Autodesk Inventor part; units mm, degrees
ref_plane "Startebene" through (0, 0, 0) normal (0, 0, 1) x (1, 0, 0)
ref_plane "Endebene" through (0, 0, 50) normal (0, 0, 1) x (1, 0, 0)
ref_plane "YZ Plane" through (0, 0, 0) normal (1, 0, 0) x (0, 1, 0)
ref_plane "Startebene" through (0, 0, 0) normal (0, 0, 1) x (1, 0, 0)
ref_plane "Endebene" through (0, 0, 50) normal (0, 0, 1) x (1, 0, 0)
sketch "Skizze2" plane through (0, 0, 0) normal (0, 0, 1) x (1, 0, 0)
  line L0 (-13.1, -4.1) -> (-13.1, 45.9)
  line L1 (-19.1, 50.9) -> (-18.1, 50.9)
  line L2 (-19.1, -19.1) -> (-19.1, 50.9)
  line L3 (-19.1, -19.1) -> (50.9, -19.1)
  line L4 (50.9, -18.1) -> (50.9, -19.1)
  line L5 (-4.1, -13.1) -> (45.9, -13.1)
  arc A0 (-13.1, -4.1) -> (-4.1, -13.1) centre (-4.1, -4.1) ccw
  arc A1 (-13.1, 45.9) -> (-18.1, 50.9) centre (-18.1, 45.9) ccw
  arc A2 (50.9, -18.1) -> (45.9, -13.1) centre (45.9, -18.1) ccw
  line L6 (0, 60.8698) -> (0, -10.145) construction
  line L7 (-10.145, 0) -> (60.8698, 0) construction
  point P0 (-13.1, -13.1)
  point P1 (-13.1, 50.9)
  point P2 (50.9, -13.1)
  dimension "d4" = 70
  dimension "d6" = 70
  dimension "d8" = 6
  dimension "d10" = 6
  dimension "d17" = 9
  dimension "d18" = 5
  dimension "d19" = 19.1
  dimension "d20" = 19.1
extrude "Körper" add sketch "Skizze2" along normal up to surface (50 mm away) from surface at 0
sketch "Sketch3" plane through (0, 0, 0) normal (0, 0, 1) x (1, 0, 0)
  line L0 (0, 0) -> (10, 0)
ref_plane "Work Plane10" through (0, 0, 0) normal (0, -1, 0) x (1, 0, 0)
sketch "Sketch4" plane through (0, 0, 0) normal (0, -1, 0) x (1, 0, 0)
  line L0 (-2, 0) -> (12, 0)
  line L1 (-2, 50) -> (12, 50)
  dimension "d24" = 50
sketch "Skizze5" plane through (-19.1, 50.9, 0) normal (-1, 0, 0) x (0, 0, 1)
  line L0 (0, -55) -> (50, -55)
  line L1 (50, -70) -> (50, 0)
  line L2 (50, -55) -> (50, 0)
  line L3 (0, 0) -> (50, 0)
  line L4 (50, 0) -> (0, 0)
  line L5 (0, -5) -> (0, -55)
  line L6 (0, 0) -> (0, -55)
  line L7 (0, -55) -> (50, -55)
  line L8 (0, -70) -> (0, 0)
  line L9 (0, 0) -> (15, 0)
  line L10 (15, 0) -> (15, -15)
  line L11 (15, -15) -> (50, -15)
  line L12 (50, -15) -> (35, -15)
  line L13 (35, -15) -> (35, -30)
  line L14 (35, -30) -> (35, -40)
  point P0 (0, -50.9)
  dimension "d25" = 15
  dimension "d26" = 15
  dimension "d27" = 15
  dimension "d28" = 15
  dimension "d29" = 10
hole "Bohrung1" at (-19.1, 35.9, 15) at (-19.1, 10.9, 35) direction (1, 0, 0) diameter 10 depth 8 tip angle 118
sketch "Skizze6" plane through (-19.1, -19.1, 0) normal (0, -1, 0) x (1, 0, 0)
  line L0 (70, 0) -> (70, 50)
  line L1 (15, 0) -> (65, 0)
  line L2 (70, 0) -> (15, 0)
  line L3 (15, 0) -> (15, 50)
  line L4 (65, 50) -> (70, 50)
  line L5 (15, 50) -> (70, 50)
  line L6 (15, 0) -> (15, 15)
  line L7 (15, 15) -> (55, 15)
  line L8 (70, 50) -> (70, 35)
  line L9 (70, 35) -> (30, 35)
  point P0 (19.1, 0)
  dimension "d37" = 15
  dimension "d38" = 40
  dimension "d39" = 15
  dimension "d40" = 40
hole "Bohrung2" at (35.9, -19.1, 15) at (10.9, -19.1, 35) direction (0, 1, 0) diameter 10 depth 8 tip angle 118
equation "\"d4\" = b"
equation "\"d6\" = b"
equation "\"d17\" = R"
equation "\"d18\" = R1"
equation "\"d19\" = ex"
equation "\"d20\" = d19"
equation "\"d11\" = G_L"
equation "\"b\" = 70"
equation "\"ParT\" = 6"
equation "\"R\" = 9"
equation "\"R1\" = 5"
equation "\"G_L\" = d24"
equation "\"ex\" = 19.1"
equation "\"G_OFFSET_START\" = 0"
equation "\"G_OFFSET_END\" = 0"
properties part number "ISO 657-1 - L70x70x6-50" material "Stahl, weich"
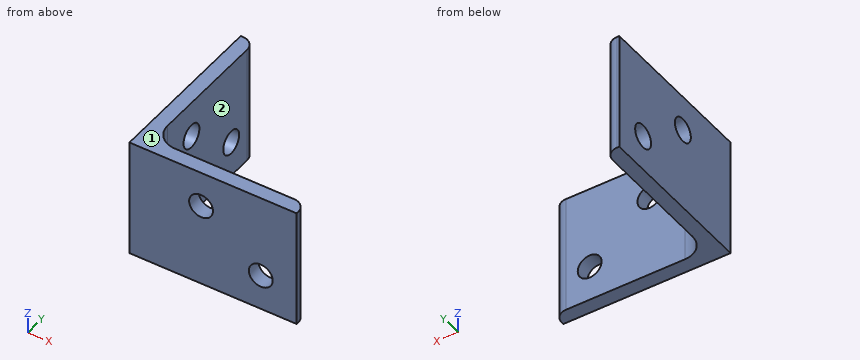
Here's how the part is built. I have some questions about the finished solid (model axes, mm). Face numbers are marked on the shaded views. A direction names the side the tool comes from. Round coordinates to 2 decimals unless told otherwise and drop trailing zeros. Loops run counter-clockwise (first coordinate to the right, second up) from the corner with the lowest first, then second, coordinate; pieces in that order, holes last.
1. For P1, Ø16, axis at y = 35.9, z = 15, coming from the -X side; P2, Ø25, axis at y = 12.5, z = 25.5, coming from the +X side; P3, Ø9, axis at x = 35.9, z = 15, coming from the -Y side; P4, Ø12, axis at x = 2, z = 40, coming from the +Y side, each with a flat end and sliding along its axis, tell me the tip position at first contact or that it passes through.
Answer list:
P1: stops at x = -19.1
P2: stops at x = -13.1
P3: passes through
P4: stops at y = -13.1
2. If we section it at D-D on z = 23.5: Write out the boundary of the cut face in (x, y).
Answer list:
outline: (-19.1, -19.1) - (50.9, -19.1) - (50.9, -18.1) arc R5 ccw to (45.9, -13.1) - (-4.1, -13.1) arc R9 cw to (-13.1, -4.1) - (-13.1, 45.9) arc R5 ccw to (-18.1, 50.9) - (-19.1, 50.9) - close
3. If I drill on line 1 along Z through (x, y) = (10.9, -15.25); line 2 along Z through (x, y) = (-14.5, 35.9); line 3 along X through (y, z) = (42, 4.5), over which ranges is the centre line in solid material (lowest first)?
Answer list:
line 1: z = 0 to 30, 40 to 50
line 2: z = 0 to 10, 20 to 50
line 3: x = -19.1 to -13.1
4. Which directions (+Z, -Z, +X, -X, +Y, -Y) give clear straight access to the entire face, cutting with the end or side of a thin tool? Please do the marked faces 1 and 2.
Answer list:
face 1: +Z, +X, -X, +Y, -Y
face 2: +Z, -Z, +X, +Y
5. If we section it at B-B on z = 15: Write out the boundary of the cut face in (x, y).
Answer list:
outline: (-19.1, -19.1) - (30.9, -19.1) - (30.9, -13.1) - (-4.1, -13.1) arc R9 cw to (-13.1, -4.1) - (-13.1, 30.9) - (-19.1, 30.9) - close; (-19.1, 40.9) - (-13.1, 40.9) - (-13.1, 45.9) arc R5 ccw to (-18.1, 50.9) - (-19.1, 50.9) - close; (40.9, -19.1) - (50.9, -19.1) - (50.9, -18.1) arc R5 ccw to (45.9, -13.1) - (40.9, -13.1) - close
6. If we section it at C-C on x = 10.9: Write out the boundary of the cut face in (y, z), plus the area to 3 significant figures.
Answer list:
outline: (-19.1, 0) - (-13.1, 0) - (-13.1, 30) - (-19.1, 30) - close; (-19.1, 40) - (-13.1, 40) - (-13.1, 50) - (-19.1, 50) - close
area: 240 mm2
7. If we section it at A-A on y = 35.9: Write out the boundary of the cut face in (x, z), plus the area to 3 significant figures.
Answer list:
outline: (-19.1, 0) - (-13.1, 0) - (-13.1, 10) - (-19.1, 10) - close; (-19.1, 20) - (-13.1, 20) - (-13.1, 50) - (-19.1, 50) - close
area: 240 mm2
